from build123d import *

# Parameters (mm, degrees)
SKETCH1_W           = 261.9375
SKETCH1_H           = 69.85
BOSS_EXTRUDE1_DEPTH = 6.35
SKETCH2_W           = 6.35
SKETCH2_H           = 38.1
CUT_EXTRUDE1_DEPTH  = 136.694110416
SCALE1_SCALE_X      = 1
SCALE1_SCALE_Y      = 1.06
SCALE1_SCALE_Z      = 1
SKETCH3_W           = 101.6
SKETCH3_H           = 19.05
CUT_EXTRUDE2_DEPTH  = 137.252717885
FILLET1_R           = 4.7625
SKETCH4_W           = 59.944
SKETCH4_H           = 2.159
BOSS_EXTRUDE2_DEPTH = 6.35


with BuildPart() as part:
    # Sketch1 → Boss-Extrude1 (new body)
    with BuildSketch(Plane.XY):
        Rectangle(SKETCH1_W, SKETCH1_H)
    extrude(amount=BOSS_EXTRUDE1_DEPTH)

    # Sketch2 → Cut-Extrude1 (cut, through all)
    with BuildSketch(Plane.XY.offset(6.35)):
        with Locations((-127.79375, -9.525)):
            Rectangle(SKETCH2_W, SKETCH2_H)
        with Locations((127.79375, -9.525)):
            Rectangle(SKETCH2_W, SKETCH2_H)
    extrude(amount=-CUT_EXTRUDE1_DEPTH, mode=Mode.SUBTRACT)


with BuildPart() as part_1:
    # Scale1: scaled about (0, 0.258743633, 3.175)
    add(part.part.scale((SCALE1_SCALE_X, SCALE1_SCALE_Y, SCALE1_SCALE_Z), about=(0, 0.258743633, 3.175)))

    # Sketch3 → Cut-Extrude2 (cut, through all)
    with BuildSketch(Plane.XY.offset(6.35)):
        with Locations((0, 27.479975382)):
            Rectangle(SKETCH3_W, SKETCH3_H)
    extrude(amount=-CUT_EXTRUDE2_DEPTH, mode=Mode.SUBTRACT)

    # Fillet1
    fillet1_edges = [part_1.edges().sort_by_distance(p)[0] for p in [
        (-124.61875, 10.080975382, 3.175),
        (-124.61875, -30.305024618, 3.175),
        (124.61875, -30.305024618, 3.175),
        (124.61875, 10.080975382, 3.175),
        (-50.8, 17.954975382, 3.175),
        (50.8, 17.954975382, 3.175),
    ]]
    fillet(fillet1_edges, radius=FILLET1_R)

    # Sketch4 → Boss-Extrude2 (add)
    with BuildSketch(Plane.XY.offset(6.35)):
        with Locations((-80.772, 38.084475382)):
            Rectangle(SKETCH4_W, SKETCH4_H)
        with Locations((80.772, 38.084475382)):
            Rectangle(SKETCH4_W, SKETCH4_H)
    extrude(amount=-BOSS_EXTRUDE2_DEPTH)


solid = part_1.part
Can you work these out from the model? Positions are in its coordinate system, mm. A direction names the side the tool comes from. Give positions to 0.01 mm unless a question says otherwise; leave off trailing zeros. Answer as a JSON object with one key per item and string values.
Q1. Will these pins go through, and if not, where does the flat tip stop? P1, Ø10, axis at x = -25, y = 23.5, coming from the +Z side; P2, Ø2, axis at y = -10, z = 3, coming from the -X side; P3, Ø3, axis at x = -3, z = 4.5, coming from the +Y side (3 decimals); P4, Ø1.7, axis at y = 38, z = 1.5, coming from the +X side.
Geometry says:
{"P1": "through", "P2": "x = -124.62", "P3": "y = 17.955", "P4": "x = 110.74"}
Q2. If I drill on L1, parallel to X at y = 29, z = 4.25; L2, parallel to Y at x = -11, z = 2; L3, parallel to X at y = -3, z = 4.25, over which ranges is the centre line in solid material (lowest first)?
Geometry says:
{"L1": "-130.97 to -50.8, 50.8 to 130.97", "L2": "-37.04 to 17.95", "L3": "-124.62 to 124.62"}
Q3. Which directions (+Z, -Z, +X, -X, +Y, -Y) give clear straight access to the entire face, cutting with the end or side of a thin tool? Please do faces 3 (the flat face through (50.8, 31, 3)), 4 (the flat face through (-81, 39.164, 3)).
Geometry says:
{"face 3": "+Z, -Z, +Y", "face 4": "+Z, -Z, +X, -X, +Y"}
Q4. If we mould it in two halves opening along X, with no side actions, what happens to faces 1 (the flat face through (-2, 2, 0)), 2 (the flat face through (-50.8, 31, 3))? For each: pulls with the +X half, pulls with the -X half, needs draft (parallel to the pull), parting line crosses it, or undercut.
Geometry says:
{"face 1": "needs draft", "face 2": "undercut"}
